```python
from build123d import *

# Parameters (mm, degrees)
SKETCH1_W           = 63.5
SKETCH1_H           = 63.5
BOSS_EXTRUDE1_DEPTH = 1.4859
CUT_EXTRUDE1_DEPTH  = 45.999517722
SKETCH3_W           = 12.7
SKETCH3_H           = 2.9718
SKETCH3_W_2         = 2.9718
SKETCH3_H_2         = 12.7
BOSS_EXTRUDE2_DEPTH = 2.9718


with BuildPart() as part:
    # Sketch1 → Boss-Extrude1 (new, symmetric)
    with BuildSketch(Plane.XY):
        Rectangle(SKETCH1_W, SKETCH1_H)
    extrude(amount=BOSS_EXTRUDE1_DEPTH, both=True)

    # Sketch2 → Cut-Extrude1 (cut, through all)
    with BuildSketch(Plane.XY.offset(1.4859)):
        Polygon((-1.524, -31.75), (-1.524, -27.94), (-3.175, -27.94), (-3.175, -25.4), (-1.524, -25.4), (-1.524, -22.225), (1.524, -22.225), (1.524, -25.4), (3.175, -25.4), (3.175, -27.94), (1.524, -27.94), (1.524, -31.75), align=None)
        Polygon((-31.75, 1.524), (-27.94, 1.524), (-27.94, 3.175), (-25.4, 3.175), (-25.4, 1.524), (-22.225, 1.524), (-22.225, -1.524), (-25.4, -1.524), (-25.4, -3.175), (-27.94, -3.175), (-27.94, -1.524), (-31.75, -1.524), align=None)
        Polygon((-1.524, 31.75), (-1.524, 27.94), (-3.175, 27.94), (-3.175, 25.4), (-1.524, 25.4), (-1.524, 22.225), (1.524, 22.225), (1.524, 25.4), (3.175, 25.4), (3.175, 27.94), (1.524, 27.94), (1.524, 31.75), align=None)
    extrude(amount=-CUT_EXTRUDE1_DEPTH, mode=Mode.SUBTRACT)

    # Sketch3 → Boss-Extrude2 (add)
    with BuildSketch(Plane.XY.offset(1.4859)):
        with Locations((-15.875, -33.2359)):
            Rectangle(SKETCH3_W, SKETCH3_H)
        with Locations((15.875, -33.2359)):
            Rectangle(SKETCH3_W, SKETCH3_H)
        with Locations((-33.2359, 15.875)):
            Rectangle(SKETCH3_W_2, SKETCH3_H_2)
        with Locations((-33.2359, -15.875)):
            Rectangle(SKETCH3_W_2, SKETCH3_H_2)
        with Locations((15.875, 33.2359)):
            Rectangle(SKETCH3_W, SKETCH3_H)
        with Locations((-15.875, 33.2359)):
            Rectangle(SKETCH3_W, SKETCH3_H)
    extrude(amount=-BOSS_EXTRUDE2_DEPTH)


solid = part.part
```
Geometry check sheet. Reference: the model listing, model coordinates, mm. A direction names the side the tool comes from. Round coordinates to 2 decimals unless told otherwise and drop trailing zeros. Loops run counter-clockwise (first coordinate to the right, second up) from the corner with the lowest first, then second, coordinate; pieces in that order, holes last. Notation, with made-up numbers: (67.5, 78.25) - (108.5, 78.25) arc R13 cw to (108.5, 89.25) - close; hole circle Ø2 at (58.5, -21). An arc over 180 degrees is marked (long way). Use a Markdown table: item, result.
Q1. Cross-section at A-A on y = 30.5. Record the cut outline in (x, z).
Solutions:
| item | result |
|---|---|
| outline | (-31.75, -1.49) - (-1.52, -1.49) - (-1.52, 1.49) - (-31.75, 1.49) - close; (1.52, -1.49) - (31.75, -1.49) - (31.75, 1.49) - (1.52, 1.49) - close |
Q2. Go/stop test with flat-tipped pins: P1, Ø1.5, axis at x = -4, z = 0, coming from the +Y side; P2, Ø0.8, axis at y = 2, z = 0, coming from the -X side; P3, Ø1.5, axis at x = -33.5, z = 0.5, coming from the +Y side (3 decimals). Record where each tip stops, or that it passes through.
Solutions:
| item | result |
|---|---|
| P1 | stops at y = 31.75 |
| P2 | stops at x = -31.75 |
| P3 | stops at y = 22.225 |
Q3. Material ranges on line 1 (Y direction, x = -2.5, z = 0.8); line 2 (X direction, y = 22.5, z = -1.1); line 3 (X direction, y = 32, z = -0.2) (3 decimals), recorded low to high.
Solutions:
| item | result |
|---|---|
| line 1 | y = -31.75 to -27.94, -25.4 to 25.4, 27.94 to 31.75 |
| line 2 | x = -31.75 to -1.52, 1.52 to 31.75 |
| line 3 | x = -22.225 to -9.525, 9.525 to 22.225 |
Q4. Cross-section at B-B on x = 27. Record the cut outline in (y, z), plus the area to 3 significant figures.
Solutions:
| item | result |
|---|---|
| outline | (-31.75, -1.49) - (31.75, -1.49) - (31.75, 1.49) - (-31.75, 1.49) - close |
| area | 189 mm2 |
Q5. Access from +Z, -Z, +X, -X, +Y, -Y to the whole of each face (thin tool, end or side, straight path). Record for faces 1 (the flat face through (-2, 25.4, 0)), 2 (the flat face through (9.525, 33, 0)), 3 (the flat face through (-24, -1.524, 0)).
Solutions:
| item | result |
|---|---|
| face 1 | +Z, -Z |
| face 2 | +Z, -Z, +Y |
| face 3 | +Z, -Z, -X |
Q6. Draft check along Y on faces 4 (the flat face through (-3.175, 27, 0)), 5 (the flat face through (0, -22.225, 0)), 6 (the flat face through (-22.225, -33, 0)). Enter one of: released by +Y, released by -Y, zero draft, split by the parting line, or undercut.
Solutions:
| item | result |
|---|---|
| face 4 | undercut |
| face 5 | released by -Y |
| face 6 | zero draft |
